The figure shows three views and two pictorial views of one solid part (mm, origin at its lowest corner). Answer the questions. Coordinates: 2 decimals unless noted, no trailing zeros. Loops run counter-clockwise (first coordinate to the right, second up) from the corner with the lowest first, then second, coordinate; pieces in that order, holes last.
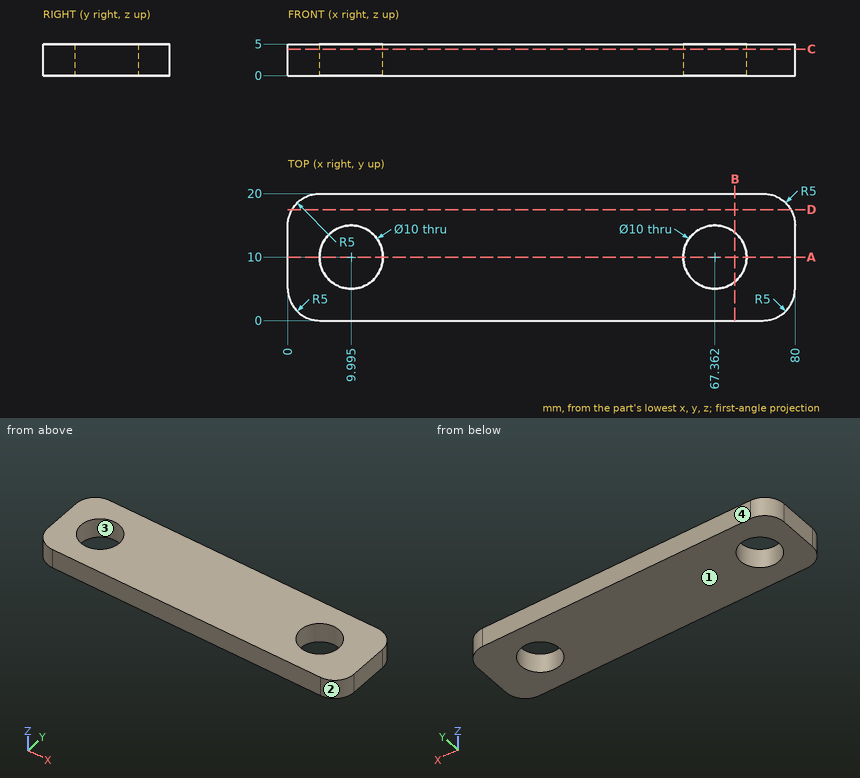
Q1. Determine the mould class of the marked faces 1, 2, 3 and 4 for opening direction Y: +Y half, -Y half, draft (parallel to the pull), parting line (faces both ways), or undercut.
Findings below:
face 1: draft
face 2: -Y half
face 3: undercut
face 4: +Y half
Q2. A cutting plane is placed at D-D (y = 17.5). Give the vertices of the cut face in (x, z), then the cut area to 3 significant figures.
Findings below:
outline: (0.67, 0) - (79.33, 0) - (79.33, 5) - (0.67, 5) - close
area: 393 mm2
Q3. A cutting plane is placed at A-A (y = 10). Give the vertices of the cut face in (x, z) (3 decimals), then the cut area to 3 significant figures.
Findings below:
outline: (0, 0) - (4.995, 0) - (4.995, 5) - (0, 5) - close; (14.995, 0) - (62.362, 0) - (62.362, 5) - (14.995, 5) - close; (72.362, 0) - (80, 0) - (80, 5) - (72.362, 5) - close
area: 300 mm2
Q4. Straight lines are drawn through the part: probe 1 along X at (y, z) = (10, 2.6) (3 decimals); probe 2 along X at (y, z) = (13, 3.8) (1 decimal); probe 3 along Y at (x, z) = (7.5, 1.15). For each, find the intervals that lie inside material, in ascending order.
Findings below:
probe 1: x = 0 to 4.995, 14.995 to 62.362, 72.362 to 80
probe 2: x = 0 to 6, 14 to 63.4, 71.4 to 80
probe 3: y = 0 to 5.67, 14.33 to 20
Q5. A cutting plane is placed at B-B (x = 70.5). Give the vertices of the cut face in (y, z).
Findings below:
outline: (0, 0) - (6.11, 0) - (6.11, 5) - (0, 5) - close; (13.89, 0) - (20, 0) - (20, 5) - (13.89, 5) - close
Q6. A cutting plane is placed at C-C (z = 4.2). Give the vertices of the cut face in (x, y) (3 decimals), then the cut area to 3 significant figures.
Findings below:
outline: (0, 5) arc R5 ccw to (5, 0) - (75, 0) arc R5 ccw to (80, 5) - (80, 15) arc R5 ccw to (75, 20) - (5, 20) arc R5 ccw to (0, 15) - close; hole circle Ø10 at (9.995, 10); hole circle Ø10 at (67.362, 10)
area: 1,420 mm2
